from build123d import *

# Parameters (mm, degrees)
SKETCH1_R            = 90
BOSS_EXTRUDE1_DEPTH  = 5
SKETCH2_W            = 90
SKETCH2_H            = 5
BOSS_EXTRUDE2_DEPTH  = 100
CUT_EXTRUDE1_DEPTH   = 100
SKETCH4_W            = 8
SKETCH4_H            = 50
CUT_EXTRUDE2_DEPTH   = 198.800404449
MIRROR2_COPY_1_DEPTH = 100
SKETCH5_W            = 5
SKETCH5_H            = 100
BOSS_EXTRUDE3_DEPTH  = 100
BOSS_EXTRUDE4_DEPTH  = 2.5
MIRROR5_COPY_1_DEPTH = 2.5
SKETCH7_R            = 3
CUT_EXTRUDE3_DEPTH   = 168.03592428
SKETCH8_R            = 4
CUT_EXTRUDE4_DEPTH   = 162.864140562


with BuildPart() as part:
    # Sketch1 → Boss-Extrude1 (new body)
    with BuildSketch(Plane(origin=(0, 0, 0), x_dir=(1, 0, 0), z_dir=(0, 1, 0))):
        with Locations(Location((0, 0, 0), (0, 0, 270))):
            Circle(SKETCH1_R)
    extrude(amount=BOSS_EXTRUDE1_DEPTH)

    # Sketch2 → Boss-Extrude2 (add)
    with BuildSketch(Plane(origin=(0, 0, 0), x_dir=(-1, 0, 0), z_dir=(0, -1, 0))):
        with Locations((0, -52.5)):
            Rectangle(SKETCH2_W, SKETCH2_H)
    boss_extrude2 = extrude(amount=BOSS_EXTRUDE2_DEPTH)

    # Sketch3 → Cut-Extrude1 (cut)
    with BuildSketch(Plane.XY.offset(55)):
        Polygon((45, -15), (9, -100), (45, -100), align=None)
    cut_extrude1 = extrude(amount=-CUT_EXTRUDE1_DEPTH, mode=Mode.SUBTRACT)

    # Mirror1: Cut-Extrude1 across plane
    add(cut_extrude1.mirror(Plane(origin=(0, 0, 0), x_dir=(0, 0, 1), z_dir=(1, 0, 0))), mode=Mode.SUBTRACT)

    # Sketch4 → Cut-Extrude2 (cut, through all)
    with BuildSketch(Plane.XY.offset(55)):
        with Locations((0, -75)):
            Rectangle(SKETCH4_W, SKETCH4_H)
    cut_extrude2 = extrude(amount=-CUT_EXTRUDE2_DEPTH, mode=Mode.SUBTRACT)

    # Mirror2: Boss-Extrude2, Cut-Extrude1, Cut-Extrude2 across plane
    add(boss_extrude2.mirror(Plane.XY))
    add(cut_extrude1.mirror(Plane.XY), mode=Mode.SUBTRACT)
    add(cut_extrude2.mirror(Plane.XY), mode=Mode.SUBTRACT)

    # Mirror2 copy 1 sketch → Mirror2 copy 1 (cut)
    with BuildSketch(Plane(origin=(0, 0, -55), x_dir=(-1, 0, 0), z_dir=(0, 0, -1))):
        Polygon((45, -15), (9, -100), (45, -100), align=None)
    extrude(amount=-MIRROR2_COPY_1_DEPTH, mode=Mode.SUBTRACT)

    # Sketch5 → Boss-Extrude3 (add)
    with BuildSketch(Plane.XZ):
        with Locations((-6.5, 0)):
            Rectangle(SKETCH5_W, SKETCH5_H)
    boss_extrude3 = extrude(amount=BOSS_EXTRUDE3_DEPTH)

    # Mirror3: Boss-Extrude3 across plane
    add(boss_extrude3.mirror(Plane(origin=(0, 0, 0), x_dir=(0, 0, 1), z_dir=(1, 0, 0))))

    # Sketch6 → Boss-Extrude4 (add, symmetric)
    with BuildSketch(Plane(origin=(-6.5, 0, 0), x_dir=(0, 0, -1), z_dir=(1, 0, 0))):
        Polygon((-55, -100), (-55, 0), (-80, 0), align=None)
    boss_extrude4 = extrude(amount=BOSS_EXTRUDE4_DEPTH, both=True)

    # Mirror4: Boss-Extrude4 across plane
    add(boss_extrude4.mirror(Plane(origin=(0, 0, 0), x_dir=(0, 0, 1), z_dir=(1, 0, 0))))

    # Mirror5: Boss-Extrude4 across plane
    add(boss_extrude4.mirror(Plane.XY))

    # Mirror5 copy 1 sketch → Mirror5 copy 1 (add, symmetric)
    with BuildSketch(Plane.ZY.offset(-6.5)):
        Polygon((-55, -100), (-55, 0), (-80, 0), align=None)
    extrude(amount=MIRROR5_COPY_1_DEPTH, both=True)

    # Sketch7 → Cut-Extrude3 (cut, through all)
    with BuildSketch(Plane(origin=(9, 0, 0), x_dir=(0, 0, -1), z_dir=(1, 0, 0))):
        with Locations((-30, -80)):
            Circle(SKETCH7_R)
    cut_extrude3 = extrude(amount=-CUT_EXTRUDE3_DEPTH, mode=Mode.SUBTRACT)

    # Mirror6: Cut-Extrude3 across plane
    add(cut_extrude3.mirror(Plane.XY), mode=Mode.SUBTRACT)

    # Sketch8 → Cut-Extrude4 (cut, through all)
    with BuildSketch(Plane.XZ):
        with Locations(Location((19, 65, 0), (0, 0, 270))):
            Circle(SKETCH8_R)
    extrude(amount=-CUT_EXTRUDE4_DEPTH, mode=Mode.SUBTRACT)


solid = part.part
Could you check a few things on this model? Use its own coordinates, in mm. A direction names the side the tool comes from. Round coordinates to 2 decimals unless told otherwise and drop trailing zeros. Write each loop counter-clockwise with the first axis right and the second up, starting at its lowest first coordinate (ties: lowest second). Pieces come first, ordered by that corner, then holes. Notation, with made-up numbers: (-37, 12.25) - (-1, 12.25) arc R19 cw to (-1, 22.25) - close; hole circle Ø3 at (89, -7). An arc over 180 degrees is marked (long way). Use a Markdown table: item, result.
Q1. I want a section at B-B (x = 0). List the corners of the cut face in (y, z) for me, plus the area to 3 significant figures.
Output values:
| item | result |
|---|---|
| outline | (-50, -55) - (0, -55) - (0, -90) - (5, -90) - (5, 90) - (0, 90) - (0, 55) - (-50, 55) - (-50, 50) - (0, 50) - (0, -50) - (-50, -50) - close |
| area | 1,400 mm2 |
Q2. For faces 4 (the flat face through (-23, -38, 55)), 5 (the flat face through (-9, -49, -1)), 6 (the flat face through (4, -49, -1)), which set-ups out of +Z, -Z, +X, -X, +Y, -Y let a thin tool reach every point of the face, with its end or its side?
Output values:
| item | result |
|---|---|
| face 4 | +Z, -X, -Y |
| face 5 | -X, -Y |
| face 6 | -Y |
Q3. I want a section at C-C (z = 65). List the corners of the cut face in (x, y) for me.
Output values:
| item | result |
|---|---|
| outline | (-62.25, 0) - (-9, 0) - (-9, -60) - (-4, -60) - (-4, 0) - (4, 0) - (4, -60) - (9, -60) - (9, 0) - (15, 0) - (15, 5) - (-62.25, 5) - close; (23, 0) - (62.25, 0) - (62.25, 5) - (23, 5) - close |
Q4. Please list where these lines run through material, in increasing order: L1, parallel to Y at x = -5.8, z = -30; L2, parallel to X at y = -90.5, z = -2.5; L3, parallel to Z at x = -0.5, y = -4.
Output values:
| item | result |
|---|---|
| L1 | -100 to -83, -77 to 5 |
| L2 | -9 to -4, 4 to 9 |
| L3 | -55 to -50, 50 to 55 |
Q5. For pin 1 (7 mm diameter, centred on y = -80, z = 30, fed in from -X); pin 2 (2.5 mm diameter, centred on x = 1, z = -51.5, fed in from -Y); pin 3 (5 mm diameter, centred on x = 15, y = -11.5, fed in from -Z); pin 4 (6 mm diameter, centred on x = 41, y = -32.5, fed in from -Z), each with a flat end and sliding along its axis, tell me the tip position at first contact or that it passes through.
Output values:
| item | result |
|---|---|
| pin 1 | x = -9 |
| pin 2 | y = -50 |
| pin 3 | z = -55 |
| pin 4 | through |
Q6. I want a section at D-D (z = 30). List the corners of the cut face in (x, y) for me.
Output values:
| item | result |
|---|---|
| outline | (-84.85, 0) - (-9, 0) - (-9, -77) - (-4, -77) - (-4, 0) - (4, 0) - (4, -77) - (9, -77) - (9, 0) - (84.85, 0) - (84.85, 5) - (-84.85, 5) - close; (-9, -100) - (-4, -100) - (-4, -83) - (-9, -83) - close; (4, -100) - (9, -100) - (9, -83) - (4, -83) - close |
Q7. Thinking about a two-plate mould opening in Z: for faces 1 (the flat face through (45, -7, 53)), 2 (the flat face through (23, -38, -50)), 3 (the flat face through (23, -38, -55)), which applies, released by +Z, released by -Z, zero draft, split by the parting line, or undercut?
Output values:
| item | result |
|---|---|
| face 1 | zero draft |
| face 2 | undercut |
| face 3 | released by -Z |
